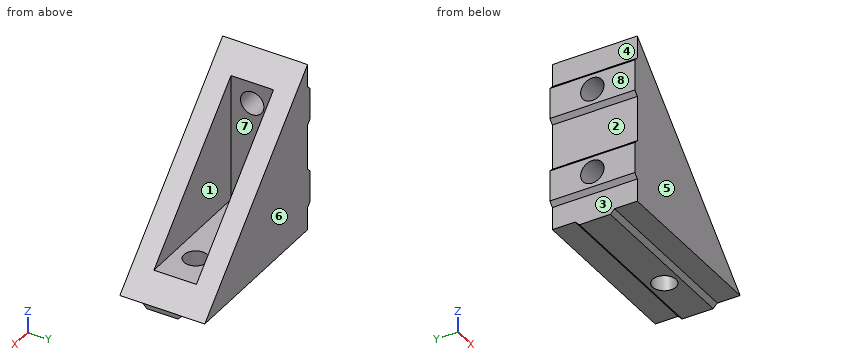
```python
from build123d import *

# Parameters (mm, degrees)
F0_W         = 40
F0_H         = 20
F1_DEPTH     = 5
F3_DEPTH     = 35
F5_DEPTH     = 40
F7_DEPTH     = 20.001
F9_DEPTH     = 20
F12_D        = 5.5
F12_ON_F11_D = 5.5


with BuildPart() as f1:
    # F0 (on Top) → F1 (new body)
    with BuildSketch(Plane.XY):
        with Locations((20, -10)):
            Rectangle(F0_W, F0_H)
    extrude(amount=F1_DEPTH)

    # F2 (on face) → F3 (join)
    with BuildSketch(Plane.XY.offset(5)):
        Polygon((0, -20), (40, -20), (40, -15), (5, -15), (5, -5), (40, -5), (40, 0), (0, 0), align=None)
    extrude(amount=F3_DEPTH)

    # F4 (on face) → F5 (join, through all)
    with BuildSketch(Plane.YZ.offset(40)):
        Polygon((-5.36, 0), (-14.64, 0), (-13.64, -1), (-6.36, -1), align=None)
    extrude(amount=-F5_DEPTH)

    # F6 (on face) → F7 (cut, through all)
    with BuildSketch(Plane.XZ.offset(20)):
        Polygon((40, 40), (0, 40), (40, 0), align=None)
    extrude(amount=-F7_DEPTH, mode=Mode.SUBTRACT)

    # F8 (on face) → F9 (join, through all)
    with BuildSketch(Plane.XZ.offset(20)):
        Polygon((0, 25.36), (0, 34.64), (-1, 33.64), (-1, 26.36), align=None)
        Polygon((0, 5.36), (0, 14.64), (-1, 13.64), (-1, 6.36), align=None)
    extrude(amount=-F9_DEPTH)

    # F12 (through all)
    with Locations(Plane.YZ.offset(5)):
        with Locations((-10, 30), (-10, 10)):
            Hole(F12_D / 2)

    # F12 on F11 (through all)
    with Locations(Plane.XY.offset(5)):
        with Locations((27, -10)):
            Hole(F12_ON_F11_D / 2)


solid = f1.part
```
For this review, take the finished solid that the model builds, in its own axes (mm). Face numbers are marked on the shaded views. A direction names the side the tool comes from. Give positions to 0.01 mm unless a question says otherwise; leave off trailing zeros. Write each loop counter-clockwise with the first axis right and the second up, starting at its lowest first coordinate (ties: lowest second). Pieces come first, ordered by that corner, then holes. Notation, with made-up numbers: M 50.5,84.25 L 82.5,84.25 A23 ccw 82.5,101.25 Z; hole C 69,54 d7. An arc over 180 degrees is marked long. Answer as CSV lines item,"result".
1. Consider section C-C, the plane z = 2. Write out the cut boundary in (x, y), then the cut area to 3 significant figures.
Findings:
outline,"M 0,-20 L 38,-20 L 38,0 L 0,0 Z; hole C 27,-10 d5.5"
area,"736 mm2"
2. Consider section A-A, the plane x = 27. Write out the cut boundary in (y, z).
Findings:
outline,"M -20,0 L -14.64,0 L -13.64,-1 L -12.75,-1 L -12.75,5 L -15,5 L -15,13 L -20,13 Z; M -7.25,-1 L -6.36,-1 L -5.36,0 L 0,0 L 0,13 L -5,13 L -5,5 L -7.25,5 Z"
3. For pin 1 (10 mm diameter, centred on y = -15.5, z = 18, fed in from +X); pin 2 (3 mm diameter, centred on y = -11, z = 1.5, fed in from -X); pin 3 (7 mm diameter, centred on y = -10, z = 30, fed in from +X); pin 4 (7 mm diameter, centred on x = 27, y = -10, fed in from -Z), all flat-tipped, find the tip position at first contact; note any pin that passes through.
Findings:
pin 1,"stops at x = 27"
pin 2,"stops at x = 0"
pin 3,"stops at x = 5"
pin 4,"stops at z = -1"
4. Draft analysis for pull direction Y (two halves, no side actions). For the marked faces 5, 6, 7 and 8, state which applies: +Y half, -Y half, draft (parallel to the pull), parting line (faces both ways), or undercut.
Findings:
face 5,"-Y half"
face 6,"+Y half"
face 7,"undercut"
face 8,"draft"
5. Wall thickness on line 1 (Y direction, x = 20, z = 17); line 2 (Z direction, x = 2.55, y = -10); line 3 (X direction, y = -8.25, z = 7): over which ranges is each line inside the solid? List them lowest first.
Findings:
line 1,"y = -20 to -15, -5 to 0"
line 2,"z = -1 to 7.25, 12.75 to 27.25, 32.75 to 37.45"
line 3,"x = -1 to 5"
6. Consider section D-D, the plane z = 10. Write out the cut boundary in (x, y).
Findings:
outline,"M -1,-20 L 30,-20 L 30,-15 L 5,-15 L 5,-12.75 L -1,-12.75 Z; M -1,-7.25 L 5,-7.25 L 5,-5 L 30,-5 L 30,0 L -1,0 Z"
7. For the marked faces 1, 2, 3 and 4, list the 3-axis set-ups (+Z, -Z, +X, -X, +Y, -Y) from which the entire face can be reached by the end or side of a thin tool; tool diameter is ignored.
Findings:
face 1,"+Z, +X"
face 2,"-X, +Y, -Y"
face 3,"-Z, -X, +Y, -Y"
face 4,"+Z, -X, +Y, -Y"
8. Consider section B-B, the plane y = -10. Write out the cut boundary in (x, z), then the cut area to 3 significant figures.
Findings:
outline,"M -1,6.36 L 0,5.36 L 0,-1 L 24.25,-1 L 24.25,5 L 5,5 L 5,7.25 L -1,7.25 Z; M -1,12.75 L 5,12.75 L 5,27.25 L -1,27.25 L -1,26.36 L 0,25.36 L 0,14.64 L -1,13.64 Z; M -1,32.75 L 5,32.75 L 5,35 L 0,40 L 0,34.64 L -1,33.64 Z; M 29.75,-1 L 40,-1 L 40,0 L 35,5 L 29.75,5 Z"
area,"308 mm2"
